```python
from build123d import *

# Parameters (mm, degrees)
F_1_8_0_125_DIAMETER_HOLE2_D = 3.175


with BuildPart() as part:
    # Sketch1 → Revolve1 (revolve)
    with BuildSketch(Plane.XY):
        Polygon((-9.525, -31.199666667), (-9.525, 13.250333333), (-23.8125, 13.250333333), (-23.8125, 6.900333333), (-12.7, 6.900333333), (-12.7, -31.199666667), align=None)
    revolve(axis=Axis((0, 0, 0), (0, 1, 0)))

    # 1/8 (0.125) Diameter Hole2 (through all)
    with Locations(Plane(origin=(0, 6.900333333, 0), x_dir=(-1, 0, 0), z_dir=(0, -1, 0))):
        with Locations((0, 19.05), (16.497783942, 9.525), (16.497783942, -9.525), (0, -19.05), (-16.497783942, -9.525), (-16.497783942, 9.525), (0, 0)):
            Hole(F_1_8_0_125_DIAMETER_HOLE2_D / 2)


solid = part.part
```
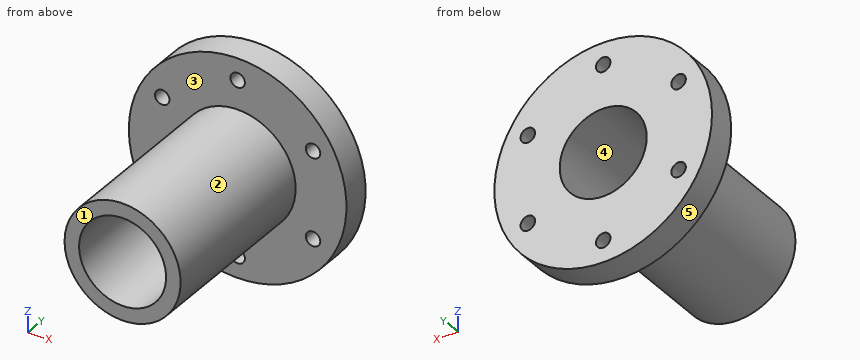
The model under review builds one solid part; all positions refer to its coordinate system, in mm. Face numbers are marked on the shaded views. A direction names the side the tool comes from. Coordinates: 2 decimals unless noted, no trailing zeros. Loops run counter-clockwise (first coordinate to the right, second up) from the corner with the lowest first, then second, coordinate; pieces in that order, holes last. Notation, with made-up numbers: (68, 57.5) -> (99, 57.5) arc R24 ccw to (99, 69.5) -> close; hole circle Ø7 at (35.25, 24.5). An arc over 180 degrees is marked (long way). Answer as CSV lines item,"result".
Item 1: Draft analysis for pull direction X (two halves, no side actions). For the marked faces 3, 4 and 5, state which applies: +X half, -X half, draft (parallel to the pull), parting line (faces both ways), or undercut.
Results below:
face 3,"draft"
face 4,"undercut"
face 5,"parting line"
Item 2: Take a section at A-A, the plane z = 0. State the section outline as (x, y) points (1 decimal), and give its area (3 significant figures).
Results below:
outline,"(-23.8, 6.9) -> (-12.7, 6.9) -> (-12.7, -31.2) -> (-9.5, -31.2) -> (-9.5, 13.3) -> (-23.8, 13.3) -> close; (9.5, -31.2) -> (12.7, -31.2) -> (12.7, 6.9) -> (23.8, 6.9) -> (23.8, 13.3) -> (9.5, 13.3) -> close"
area,"423 mm2"
Item 3: Take a section at B-B, the plane x = 0. State the section outline as (y, z) points (1 decimal), and give its area (3 significant figures).
Results below:
outline,"(-31.2, -12.7) -> (6.9, -12.7) -> (6.9, -17.5) -> (13.3, -17.5) -> (13.3, -9.5) -> (-31.2, -9.5) -> close; (-31.2, 9.5) -> (13.3, 9.5) -> (13.3, 17.5) -> (6.9, 17.5) -> (6.9, 12.7) -> (-31.2, 12.7) -> close; (6.9, -23.8) -> (13.3, -23.8) -> (13.3, -20.6) -> (6.9, -20.6) -> close; (6.9, 20.6) -> (13.3, 20.6) -> (13.3, 23.8) -> (6.9, 23.8) -> close"
area,"383 mm2"
Item 4: Machinability: for the marked faces 1 and 2, which of the approach directions +Z, -Z, +X, -X, +Y, -Y give a long, thin tool a straight path to every point of the face, cutting with its end or side? Answer none if there is none.
Results below:
face 1,"+Z, -Z, +X, -X, -Y"
face 2,"-Y"
Item 5: For L1, parallel to Z at x = 0, y = 12 (1 decimal); L2, parallel to Z at x = 0, y = -18 (3 decimals); L3, parallel to Y at x = -1, z = 13, list the stretches that pass through material, from the lowest coordinate up.
Results below:
L1,"z = -23.8 to -20.6, -17.5 to -9.5, 9.5 to 17.5, 20.6 to 23.8"
L2,"z = -12.7 to -9.525, 9.525 to 12.7"
L3,"y = 6.9 to 13.25"
Item 6: Take a section at D-D, the plane y = 5.5. State the section outline as (x, z) points (3 decimals), and give its area (3 significant figures).
Results below:
outline,"circle Ø25.4 at (0, 0); hole circle Ø19.05 at (0, 0)"
area,"222 mm2"
Item 7: Insertion check: pin 1 (1 mm diameter, centred on x = -10, y = -4.5, fed in from +Z); pin 2 (8 mm diameter, centred on y = -13.5, z = 14, fed in from -X); pin 3 (5 mm diameter, centred on x = 16.5, z = -9.52, fed in from -Y); pin 4 (1.9 mm diameter, centred on x = 0, z = 19.05, fed in from +Y). Each pin has a flat end and moves straight along its axis. Give the tip position at first contact, or say it passes through.
Results below:
pin 1,"stops at z = 8.43"
pin 2,"stops at x = -7.83"
pin 3,"stops at y = 6.9"
pin 4,"passes through"
Item 8: Take a section at C-C, the plane x = -16. State the section outline as (y, z) points.
Results below:
outline,"(6.9, -17.64) -> (13.25, -17.64) -> (13.25, -11.03) -> (6.9, -11.03) -> close; (6.9, -8.02) -> (13.25, -8.02) -> (13.25, 8.02) -> (6.9, 8.02) -> close; (6.9, 11.03) -> (13.25, 11.03) -> (13.25, 17.64) -> (6.9, 17.64) -> close"
